CAD build for the part. Positions are in the model's coordinates, mm. A direction names the side the tool comes from. Round coordinates to 2 decimals unless told otherwise and drop trailing zeros. Write each loop counter-clockwise with the first axis right and the second up, starting at its lowest first coordinate (ties: lowest second). Pieces come first, ordered by that corner, then holes. Notation, with made-up numbers: (82, -16.75) - (125, -16.75) arc R20 cw to (125, 20.25) - close; hole circle Ø4 at (77, -39). An arc over 180 degrees is marked (long way). Answer in a Markdown table with one row per item.
```python
from build123d import *

# Parameters (mm, degrees)
SKETCH_1_W          = 350
SKETCH_1_H          = 50
SKETCH_1_R          = 4
EXTRUDE_1_DEPTH     = 10
EXTRUDE_2_DEPTH     = 50
CUT_EXTRUDE_1_DEPTH = 20
CUT_EXTRUDE_2_DEPTH = 20
SKETCH_5_R          = 6
CUT_EXTRUDE_3_DEPTH = 20
SKETCH_6_R          = 9
CUT_EXTRUDE_4_DEPTH = 4


with BuildPart() as part:
    # 草图1 → 凸台-拉伸1 (new body)
    with BuildSketch(Plane(origin=(0, 0, 0), x_dir=(1, 0, 0), z_dir=(0, 1, 0))):
        with Locations((175, 25)):
            Rectangle(SKETCH_1_W, SKETCH_1_H)
        with Locations(Location((15, 25, 0), (0, 0, 270))):
            Circle(SKETCH_1_R, mode=Mode.SUBTRACT)
        with Locations(Location((335, 25, 0), (0, 0, 90))):
            Circle(SKETCH_1_R, mode=Mode.SUBTRACT)
    extrude(amount=EXTRUDE_1_DEPTH)

    # 草图2 → 凸台-拉伸2 (add)
    with BuildSketch(Plane.XY):
        Polygon((170.81786786, 65.231720812), (152.463883228, 207.062743075), (162.381189023, 208.346115889), (188.0486453, 10), (175, 10), (133, 10), align=None)
    extrude(amount=-EXTRUDE_2_DEPTH)

    # 草图3 → 切除-拉伸1 (cut)
    with BuildSketch(Plane.XY):
        Polygon((177.96526156, 10), (133, 10), (170.81786786, 65.231720812), align=None)
    extrude(amount=-CUT_EXTRUDE_1_DEPTH, mode=Mode.SUBTRACT)

    # 草图4 → 切除-拉伸2 (cut)
    with BuildSketch(Plane(origin=(0, 0, -50), x_dir=(-1, 0, 0), z_dir=(0, 0, -1))):
        Polygon((-170.81786786, 65.231720812), (-177.96526156, 10), (-133, 10), align=None)
    extrude(amount=-CUT_EXTRUDE_2_DEPTH, mode=Mode.SUBTRACT)

    # 草图5 → 切除-拉伸3 (cut)
    with BuildSketch(Plane(origin=(186.224158089, 24.098785167, 0), x_dir=(0, 0, -1), z_dir=(0.9917305794448423, 0.12833728138774617, 0))):
        with Locations(Location((25, 95.783653888, 0), (0, 0, 90))):
            Circle(SKETCH_5_R)
        with Locations(Location((25, 155.783653888, 0), (0, 0, 90))):
            Circle(SKETCH_5_R)
    extrude(amount=-CUT_EXTRUDE_3_DEPTH, mode=Mode.SUBTRACT)

    # 草图6 → 切除-拉伸4 (cut)
    with BuildSketch(Plane(origin=(176.306852295, 22.815412353, 0), x_dir=(0, 0, 1), z_dir=(-0.9917305794448422, -0.1283372813877468, 0))):
        with Locations(Location((-25, 155.783653888, 0), (0, 0, 270))):
            Circle(SKETCH_6_R)
        with Locations(Location((-25, 95.783653888, 0), (0, 0, 270))):
            Circle(SKETCH_6_R)
    extrude(amount=-CUT_EXTRUDE_4_DEPTH, mode=Mode.SUBTRACT)


solid = part.part
```
Q1. Saw through at C-C on x = 275. List the corners of the cut face in (y, z), then the cut area to 3 significant figures.
Computed:
| item | result |
|---|---|
| outline | (0, -50) - (10, -50) - (10, 0) - (0, 0) - close |
| area | 500 mm2 |
Q2. Flat gauge pins, fed straight in: pin 1 (13.5 mm diameter, centred on x = 150.5, y = 26.5, fed in from +Z); pin 2 (1 mm diameter, centred on y = 174, z = -15, fed in from +X); pin 3 (25 mm diameter, centred on x = 300, z = -17.5, fed in from +Y); pin 4 (6 mm diameter, centred on x = 169.5, z = -22.5, fed in from -Y). Where does each tip first touch, or does it go through?
Computed:
| item | result |
|---|---|
| pin 1 | stops at z = -20 |
| pin 2 | stops at x = 166.89 |
| pin 3 | stops at y = 10 |
| pin 4 | stops at y = 0 |
Q3. Saw through at D-D on y = 74. List the corners of the cut face in (x, z).
Computed:
| item | result |
|---|---|
| outline | (169.68, -50) - (179.77, -50) - (179.77, 0) - (169.68, 0) - close |
Q4. Pull direction Z, two halves, no side cores. Call faces 4 (the flat face through (0, 5, -25)), 5 (the flat face through (160.52, 175.97, -30.87)), 6 (the flat face through (174, 50, 0)), 7 (the flat face through (168.22, 116.46, -30.87)): released by +Z, released by -Z, zero draft, split by the parting line, or undercut.
Computed:
| item | result |
|---|---|
| face 4 | zero draft |
| face 5 | undercut |
| face 6 | released by +Z |
| face 7 | undercut |
Q5. Saw through at A-A on x = 15. List the corners of the cut face in (y, z).
Computed:
| item | result |
|---|---|
| outline | (0, -50) - (10, -50) - (10, -29) - (0, -29) - close; (0, -21) - (10, -21) - (10, 0) - (0, 0) - close |
Q6. Saw through at B-B on z = -11. List the corners of the cut face in (x, y), then the cut area to 3 significant figures.
Computed:
| item | result |
|---|---|
| outline | (0, 0) - (350, 0) - (350, 10) - (188.05, 10) - (162.38, 208.35) - (152.46, 207.06) - (177.97, 10) - (0, 10) - close |
| area | 5,490 mm2 |
Q7. Drill centre lines: line 1 (X direction, y = 6.75, z = -25); line 2 (Z direction, x = 335, y = 7.25); line 3 (Y direction, x = 255, z = -29). Where is each one in solid material? Low to high.
Computed:
| item | result |
|---|---|
| line 1 | x = 0 to 11, 19 to 331, 339 to 350 |
| line 2 | z = -50 to -29, -21 to 0 |
| line 3 | y = 0 to 10 |
Q8. 3-axis set-ups, long thin cutter, end or side, ignore diameter. For faces 1 (the flat face through (161, 32, -30)), 2 (the flat face through (151.644, 37.229, -24.93)), 3 (the flat face through (161, 32, -20)): which of +Z, -Z, +X, -X, +Y, -Y reach the whole face in a straight line?
Computed:
| item | result |
|---|---|
| face 1 | -Z, -X |
| face 2 | +Z, -Z, -X |
| face 3 | +Z, -X |
